Study the drawing (mm; zero at the part's minimum x, y, z) and answer. A direction names the side the tool comes from. Coordinates: 2 decimals unless noted, no trailing zeros. Loops run counter-clockwise (first coordinate to the right, second up) from the corner with the lowest first, then second, coordinate; pieces in that order, holes last. Notation, with made-up numbers: (29, 87) - (42, 87) arc R15 cw to (42, 116) - close; hole circle Ø11 at (58.25, -34.5). An arc over 180 degrees is marked (long way). Put each result on its own line as item: value.
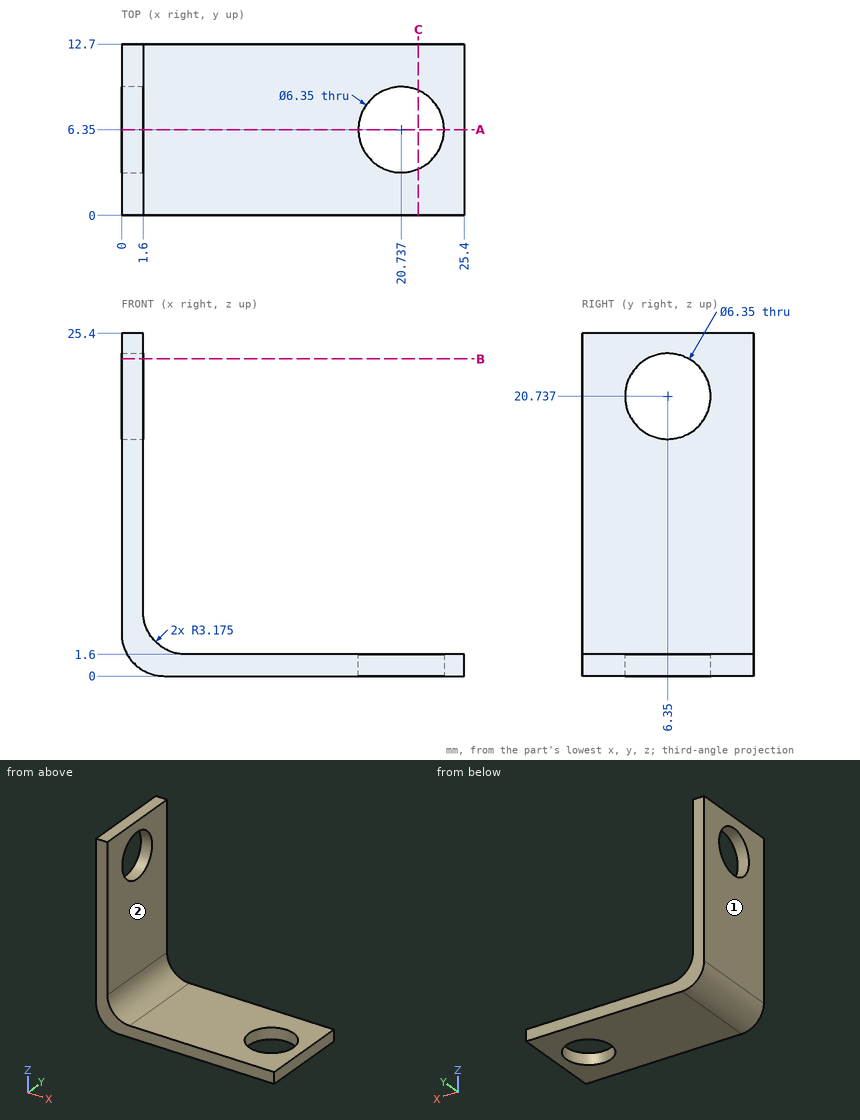
1) The part is cut by section A-A (y = 6.35). State how many separate pieces and enclosed holes the cut face has.
Found:
separate pieces: 3
enclosed holes: 0
2) The part is cut by section C-C (x = 22). Give the vertices of the cut face in (y, z), and give its area (3 significant figures).
Found:
outline: (0, 0) - (3.44, 0) - (3.44, 1.6) - (0, 1.6) - close; (9.26, 0) - (12.7, 0) - (12.7, 1.6) - (9.26, 1.6) - close
area: 11.0 mm^2
3) Straight lines are drawn through the part: L1, parallel to Z at x = 13, y = 3.75; L2, parallel to X at y = 9, z = 1 (1 decimal); L3, parallel to Z at x = 0.75, y = 6.35 (1 decimal). For each, find the intervals that lie inside material, in ascending order. Write a range as [from, to].
Found:
L1: z = [0, 1.6]
L2: x = [0.9, 19], [22.5, 25.4]
L3: z = [1.1, 17.6], [23.9, 25.4]
4) Each of these flat-tipped pins is pushed along its axis until it touches: pin 1 (3 mm diameter, centred on x = 11, y = 11, fed in from +Z); pin 2 (12 mm diameter, centred on x = 9.5, z = 13, fed in from +Y). Where does it stop, or does it pass through?
Found:
pin 1: stops at z = 1.6
pin 2: passes through
5) The part is cut by section B-B (z = 23.5). Give the vertices of the cut face in (x, y).
Found:
outline: (0, 0) - (1.6, 0) - (1.6, 4.79) - (0, 4.79) - close; (0, 7.91) - (1.6, 7.91) - (1.6, 12.7) - (0, 12.7) - close
6) For the marked faces 1 and 2, determine the directions among +Z, -Z, +X, -X, +Y, -Y from which every point of the face is accessible in a straight line to the end or side of a thin tool.
Found:
face 1: +Z, -Z, -X, +Y, -Y
face 2: +Z, +X, +Y, -Y
